Check sheet for the modelled part. Datum: model origin and axes. Units: mm. Round coordinates to 2 decimals unless told otherwise and drop trailing zeros. Order: outer loops, then holes, each group sorted by start corner. A loop starts at its lowest first (then second) coordinate and runs counter-clockwise, first axis right, second up. Notation, with made-up numbers: (-18.5, -19.5) -> (15.5, -19.5) arc R20 cw to (15.5, -6.5) -> close; hole circle Ø3 at (0, -3). An arc over 180 degrees is marked (long way). Use CSV: the item, a comma, the result in double quotes.
```python
from build123d import *

# Parameters (mm, degrees)
BOSS_EXTRUDE1_DEPTH      = 14
FILLET1_R                = 2.54
FILLET2_R                = 2.54
F_9_16_18_TAPPED_HOLE1_D = 13.09624


with BuildPart() as part:
    # Sketch1 → Boss-Extrude1 (new body)
    with BuildSketch(Plane.XY):
        with BuildLine():
            Line((-80, -15), (53.524252006, -15))
            ThreePointArc((53.524252006, -15), (70.333541706, -15.696449958), (87.02760671, -17.78102579))
            ThreePointArc((87.02760671, -17.78102579), (108.027756377, 0), (87.02760671, 17.78102579))
            ThreePointArc((87.02760671, 17.78102579), (70.333541706, 15.696449958), (53.524252006, 15))
            Line((53.524252006, 15), (-80, 15))
            Line((-80, 15), (-80, -15))
        make_face()
    extrude(amount=BOSS_EXTRUDE1_DEPTH)

    # Fillet1
    fillet1_edges = [part.edges().sort_by_distance(p)[0] for p in [
        (70.333541706, -15.696449958, 14),
        (108.027756377, 0, 14),
        (70.333541706, 15.696449958, 14),
        (-13.237873997, 15, 14),
        (-80, 0, 14),
        (-13.237873997, -15, 14),
    ]]
    fillet(fillet1_edges, radius=FILLET1_R)

    # Fillet2
    fillet2_edges = [part.edges().sort_by_distance(p)[0] for p in [
        (-13.237873997, 15, 0),
        (70.333541706, 15.696449958, 0),
        (108.027756377, 0, 0),
        (70.333541706, -15.696449958, 0),
        (-13.237873997, -15, 0),
        (-80, 0, 0),
    ]]
    fillet(fillet2_edges, radius=FILLET2_R)

    # 9/16-18 Tapped Hole1 (through all)
    with Locations(Plane.XY.offset(14)):
        with Locations((90, 0)):
            Hole(F_9_16_18_TAPPED_HOLE1_D / 2)


solid = part.part
```
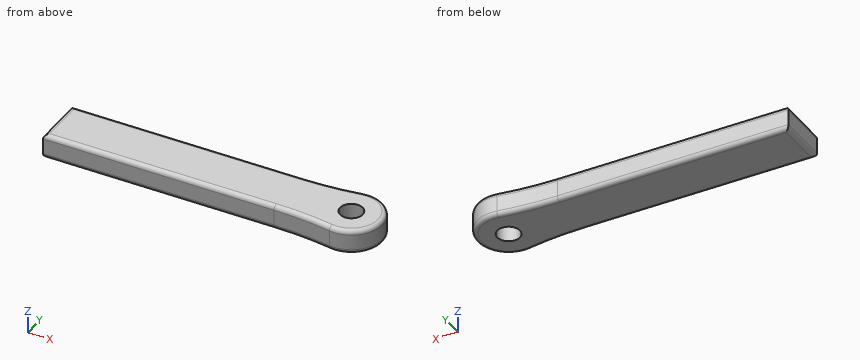
Q1. Sectioned sample at B-B, the plane z = 7.5. Enter the section's corners in (x, y).
Result sheet:
outline,"(-80, -15) -> (53.52, -15) arc R203.2 cw to (87.03, -17.78) arc R18.03 ccw (long way) to (87.03, 17.78) arc R203.2 cw to (53.52, 15) -> (-80, 15) -> close; hole circle Ø13.1 at (90, 0)"
Q2. Sectioned sample at A-A, the plane y = 0. Enter the section's corners in (x, z), then the cut area to 3 significant figures.
Result sheet:
outline,"(-80, 2.54) arc R2.54 ccw to (-77.46, 0) -> (83.45, 0) -> (83.45, 14) -> (-77.46, 14) arc R2.54 ccw to (-80, 11.46) -> close; (96.55, 0) -> (105.49, 0) arc R2.54 ccw to (108.03, 2.54) -> (108.03, 11.46) arc R2.54 ccw to (105.49, 14) -> (96.55, 14) -> close"
area,"2,440 mm^2"
Q3. Go/stop test with flat-tipped pins: pin 1 (4 mm diameter, centred on x = 12.5, z = 12.5, fed in from -Y); pin 2 (10.5 mm diameter, centred on x = 90, y = 0, fed in from +Z) (1 decimal); pin 3 (8 mm diameter, centred on y = -13.5, z = 2.5, fed in from +X); pin 4 (4 mm diameter, centred on x = 17, z = 11, fed in from +Y). Record where each tip stops, or that it passes through.
Result sheet:
pin 1,"stops at y = -15"
pin 2,"passes through"
pin 3,"stops at x = 105.32"
pin 4,"stops at y = 15"
Q4. Sectioned sample at C-C, the plane x = -4.5. Enter the section's corners in (y, z), then the cut area to 3 significant figures.
Result sheet:
outline,"(-15, 2.54) arc R2.54 ccw to (-12.46, 0) -> (12.46, 0) arc R2.54 ccw to (15, 2.54) -> (15, 11.46) arc R2.54 ccw to (12.46, 14) -> (-12.46, 14) arc R2.54 ccw to (-15, 11.46) -> close"
area,"414 mm^2"
Q5. Scan lines: L1, parallel to Y at x = 90, z = 9.25; L2, parallel to Y at x = 6, z = 7.5; L3, parallel to X at y = -4.5, z = 7.75. Record each from-to range of solid material in increasing order.
Result sheet:
L1,"y = -18.03 to -6.55, 6.55 to 18.03"
L2,"y = -15 to 15"
L3,"x = -80 to 85.24, 94.76 to 107.46"
